Build history of the part. All positions in model axes, mm. A direction names the side the tool comes from. Give positions to 0.01 mm unless a question says otherwise; leave off trailing zeros. Write each loop counter-clockwise with the first axis right and the second up, starting at its lowest first coordinate (ties: lowest second). Pieces come first, ordered by that corner, then holes. Notation, with made-up numbers: (41, -39.75) -> (100, -39.75) arc R14 ccw to (100, -30.75) -> close; hole circle Ø5 at (-34, 39). An arc over 180 degrees is marked (long way). Put each result on its own line as item: value. Start each with the question number.
Item 1: Two-plate mould, pull along Z, no slides. Class faces 1 (the cylindrical face through (-248.83, 40.496, -310.566)), 2 (the conical face through (-92.495, 127.545, -293.713)), 3 (the flat face through (-182, 150, -224)), 4 (the cylindrical face through (-125.421, 40.496, 367.003)): pulls with the +Z half, pulls with the -Z half, needs draft (parallel to the pull), parting line crosses it, or undercut.
Item 2: Tool access for faces 5 (the flat face through (97, 5, -365)), 6 (the cylindrical face through (127.355, 40.496, 367.003)), 7 (the cylindrical face through (297.552, 140.14, 66.075)): list every direction of +Z, -Z, +X, -X, +Y, -Y with a clear straight run to the whole face (end or side of a thin tool).
Item 3: Slice it at A-A, the plane x = 0. List the corners of the cut face in (y, z), plus the area to 3 significant figures.
Item 4: Flat gauge pins, fed straight in: pin 1 Ø2 at (x, y) = (39, 19.5) entering from -Z; pin 2 Ø3 at (x, y) = (123, 132.5) entering from +Z; pin 3 Ø5 at (x, z) = (-338.5, 211.5) entering from -Y. Where does each tip first touch, or does it go through?
Item 5: Slice it at B-B, the plane y = 61. Give the number of separate pieces and of enclosed holes in the cut face, plus the area to 3 significant figures.
Item 6: Drill centre lines: line 1 along X through (y, z) = (48, 0); line 2 along Z through (x, y) = (2, 16.5); line 3 along X through (y, z) = (7, 232.5). Where is each one in solid material? Low to high.
```python
from build123d import *

# Parameters (mm, degrees)
SKETCH2_R          = 22
CUT_EXTRUDE2_DEPTH = 270


with BuildPart() as part:
    # Sketch1 → Revolve2 (revolve)
    with BuildSketch(Plane.XY, mode=Mode.PRIVATE) as revolve2_sk:
        with BuildLine():
            Line((445, 77), (375, 77))
            ThreePointArc((375, 77), (372.006131672, 77.84404461), (369.329788537, 79.429240589))
            Line((369.329788537, 79.429240589), (304.8, 130))
            Line((304.8, 130), (304.8, 150))
            Line((304.8, 150), (287.4, 150))
            Line((287.4, 150), (287.4, 0))
            Line((287.4, 0), (370, 0))
            Line((370, 0), (375, 5))
            Line((375, 5), (445, 5))
            Line((445, 5), (445, 77))
        make_face()
    revolve(revolve2_sk.sketch.rotate(Axis((0, 92.097125436, 0), (0, 1, 0)), 90), axis=Axis((0, 92.097125436, 0), (0, 1, 0)))

    # Sketch2 → Cut-Extrude2 (cut, symmetric)
    with BuildSketch(Plane(origin=(0, 0, 0), x_dir=(1, 0, 0), z_dir=(0, 1, 0))):
        with Locations(Location((409, 0, 0), (0, 0, 270))):
            Circle(SKETCH2_R)
        with Locations(Location((388.982115165, -126.387950699, 0), (0, 0, 270))):
            Circle(SKETCH2_R)
        with Locations(Location((330.887950699, -240.404168188, 0), (0, 0, 270))):
            Circle(SKETCH2_R)
        with Locations(Location((240.404168188, -330.887950699, 0), (0, 0, 270))):
            Circle(SKETCH2_R)
        with Locations(Location((126.387950699, -388.982115165, 0), (0, 0, 270))):
            Circle(SKETCH2_R)
        with Locations(Location((0, -409, 0), (0, 0, 270))):
            Circle(SKETCH2_R)
        with Locations(Location((-126.387950699, -388.982115165, 0), (0, 0, 270))):
            Circle(SKETCH2_R)
        with Locations(Location((-240.404168188, -330.887950699, 0), (0, 0, 270))):
            Circle(SKETCH2_R)
        with Locations(Location((-330.887950699, -240.404168188, 0), (0, 0, 270))):
            Circle(SKETCH2_R)
        with Locations(Location((-388.982115165, -126.387950699, 0), (0, 0, 270))):
            Circle(SKETCH2_R)
        with Locations(Location((-409, 0, 0), (0, 0, 270))):
            Circle(SKETCH2_R)
        with Locations(Location((-388.982115165, 126.387950699, 0), (0, 0, 270))):
            Circle(SKETCH2_R)
        with Locations(Location((-330.887950699, 240.404168188, 0), (0, 0, 270))):
            Circle(SKETCH2_R)
        with Locations(Location((-240.404168188, 330.887950699, 0), (0, 0, 270))):
            Circle(SKETCH2_R)
        with Locations(Location((-126.387950699, 388.982115165, 0), (0, 0, 270))):
            Circle(SKETCH2_R)
        with Locations(Location((0, 409, 0), (0, 0, 270))):
            Circle(SKETCH2_R)
        with Locations(Location((126.387950699, 388.982115165, 0), (0, 0, 270))):
            Circle(SKETCH2_R)
        with Locations(Location((240.404168188, 330.887950699, 0), (0, 0, 270))):
            Circle(SKETCH2_R)
        with Locations(Location((330.887950699, 240.404168188, 0), (0, 0, 270))):
            Circle(SKETCH2_R)
        with Locations(Location((388.982115165, 126.387950699, 0), (0, 0, 270))):
            Circle(SKETCH2_R)
    extrude(amount=CUT_EXTRUDE2_DEPTH, both=True, mode=Mode.SUBTRACT)


solid = part.part
```
Values follow:
1. face 1: undercut
1. face 2: parting line crosses it
1. face 3: needs draft
1. face 4: undercut
2. face 5: -Y
2. face 6: +Y, -Y
2. face 7: +Y
3. outline: (0, -370) -> (5, -375) -> (5, -387) -> (77, -387) -> (77, -375) arc R12 cw to (79.43, -369.33) -> (130, -304.8) -> (150, -304.8) -> (150, -287.4) -> (0, -287.4) -> close; (0, 287.4) -> (150, 287.4) -> (150, 304.8) -> (130, 304.8) -> (79.43, 369.33) arc R12 cw to (77, 375) -> (77, 387) -> (5, 387) -> (5, 375) -> (0, 370) -> close; (5, -445) -> (77, -445) -> (77, -431) -> (5, -431) -> close; (5, 431) -> (77, 431) -> (77, 445) -> (5, 445) -> close
3. area: 23,300 mm2
4. pin 1: z = -443.37
4. pin 2: z = 279.54
4. pin 3: y = 5
5. separate pieces: 1
5. enclosed holes: 21
5. area: 332,000 mm2
6. line 1: -445 to -431, -387 to -287.4, 287.4 to 387, 431 to 445
6. line 2: -445 to -430.91, -387.09 to -287.39, 287.39 to 387.09, 430.91 to 445
6. line 3: -379.43 to -351.42, -310.36 to -168.95, 168.95 to 310.36, 351.42 to 379.43
